Build history of the part. All positions in model axes, mm. A direction names the side the tool comes from. Coordinates: 2 decimals unless noted, no trailing zeros. Loops run counter-clockwise (first coordinate to the right, second up) from the corner with the lowest first, then second, coordinate; pieces in that order, holes last.
Item 1: 3-axis set-ups, long thin cutter, end or side, ignore diameter. For faces 1 (the face through (-300, -4, 493)), 2 (the face through (2, -75, 1074)), 3 (the face through (150, 1, 1074)), 4 (the face through (-2, 75, 1074)), 5 (the face through (-150, -1, 1074)): which of +Z, -Z, +X, -X, +Y, -Y reach the whole face in a straight line?
Item 2: Cut at A-A (x = 96.5). List the corners of the cut face in (y, z).
Item 3: Drill centre lines: line 1 along Y through (x, z) = (51.5, 1010); line 2 along Z through (x, y) = (-216, 218.5). Where is each one in solid material? Low to high.
Item 4: Flat gauge pin, fed straight in: pin 1 (3 mm diameter, centred on x = -199, y = -177, fed in from +Z). Where does the tip first touch, or does it go through?
Item 5: Cut at B-B (y = -234.5). List the corners of the cut face in (x, z).
Autodesk Inventor part; units mm, degrees
ref_plane "YZ Plane" through (0, 0, 0) normal (1, 0, 0) x (0, 1, 0)
ref_plane "XZ Plane" through (0, 0, 0) normal (0, 1, 0) x (-1, 0, 0)
ref_plane "XY Plane" through (0, 0, 0) normal (0, 0, 1) x (1, 0, 0)
sketch "Sketch1" plane through (0, 0, 0) normal (0, 0, 1) x (1, 0, 0)
  line L0 (-300, 300) -> (300, 300)
  line L1 (300, 300) -> (300, -300)
  line L2 (300, -300) -> (-300, -300)
  line L3 (-300, -300) -> (-300, 300)
  line L4 (-300, -300) -> (300, 300) construction
  point P0 (0, 0)
  point P1 (0, 0)
  dimension "d0" = 600
  dimension "d1" = 600
extrude "Extrusion1" add sketch "Sketch1" along normal blind 1000
sketch "Sketch2" plane through (0, 0, 1000) normal (0, 0, 1) x (1, 0, 0)
  line L0 (-150, 75) -> (150, 75)
  line L1 (150, 75) -> (150, -75)
  line L2 (150, -75) -> (-150, -75)
  line L3 (-150, -75) -> (-150, 75)
  line L4 (-150, 75) -> (150, -75) construction
  line L5 (150, 75) -> (-150, -75) construction
  point P0 (0, 0)
  dimension "d4" = 300
  dimension "d5" = 150
extrude "Extrusion2" add sketch "Sketch2" along normal blind 150
equation "\"d0\" = Длина"
equation "\"d1\" = Ширина"
equation "\"d2\" = Высота"
equation "\"Длина\" = 600"
equation "\"Ширина\" = 600"
equation "\"Высота\" = 1000"
properties part number "Coagulant barrel"
Filled sheet:
1. face 1: +Z, -Z, -X, +Y, -Y
1. face 2: +Z, +X, -X, -Y
1. face 3: +Z, +X, +Y, -Y
1. face 4: +Z, +X, -X, +Y
1. face 5: +Z, -X, +Y, -Y
2. outline: (-300, 0) - (300, 0) - (300, 1000) - (75, 1000) - (75, 1150) - (-75, 1150) - (-75, 1000) - (-300, 1000) - close
3. line 1: y = -75 to 75
3. line 2: z = 0 to 1000
4. pin 1: stops at z = 1000
5. outline: (-300, 0) - (300, 0) - (300, 1000) - (-300, 1000) - close
